The figure shows three views and two pictorial views of one solid part (mm, origin at its lowest corner). Answer the questions. A direction names the side the tool comes from. Coordinates: 2 decimals unless noted, no trailing zeros. Loops run counter-clockwise (first coordinate to the right, second up) from the corner with the lowest first, then second, coordinate; pieces in that order, holes last.
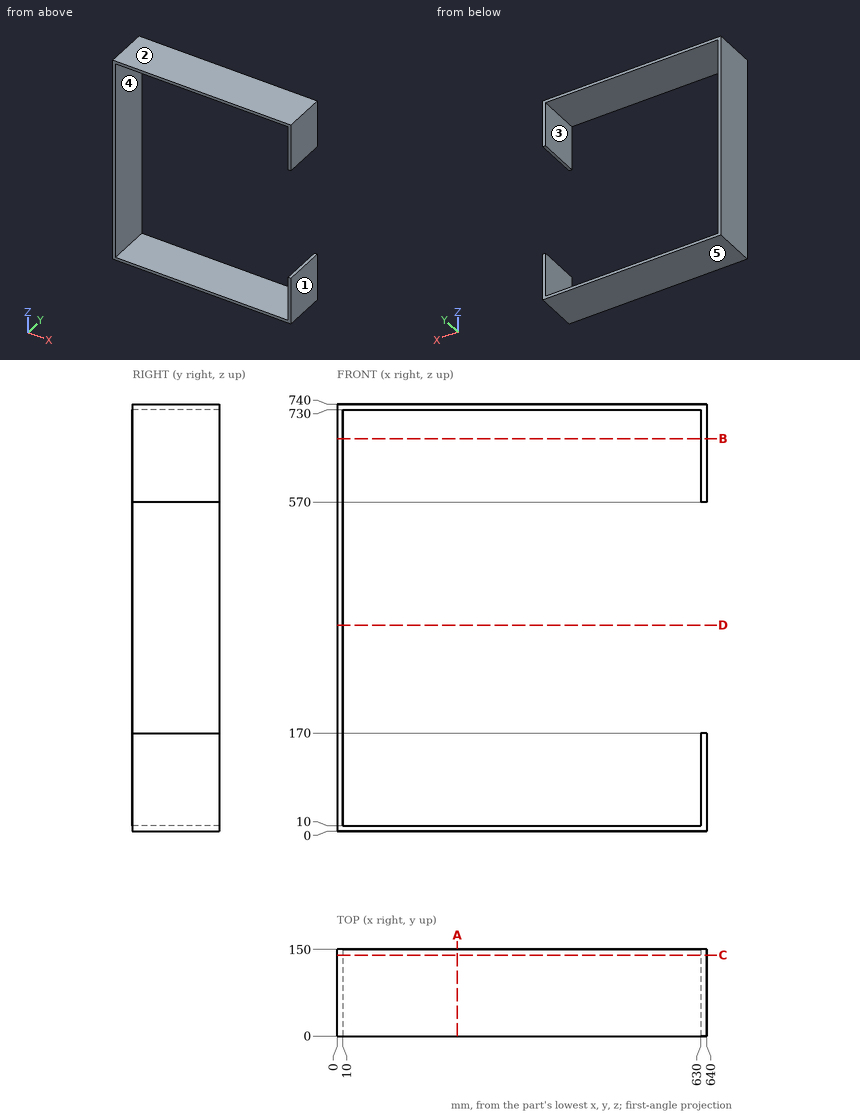
Q1. A cutting plane is placed at A-A (x = 208.5). Give the vertices of the cut face in (y, z), then the cut area to 3 significant figures.
Findings below:
outline: (0, 0) - (150, 0) - (150, 10) - (0, 10) - close; (0, 730) - (150, 730) - (150, 740) - (0, 740) - close
area: 3,000 mm2
Q2. A flat-ended cylindrical pin translates along its axis: pin 1 Ø3 at (y, z) = (65.5, 269) entering from +X. Find the tip coordinate at first contact, or state that the pin passes through.
Findings below:
pin 1: stops at x = 10
Q3. Determine the mould class of the marked faces 1, 2 and 3 for opening direction X: +X half, -X half, draft (parallel to the pull), parting line (faces both ways), or undercut.
Findings below:
face 1: +X half
face 2: draft
face 3: undercut
Q4. A cutting plane is placed at D-D (z = 357). Give the vertices of the cut face in (x, y), then the cut area to 3 significant figures.
Findings below:
outline: (0, 0) - (10, 0) - (10, 150) - (0, 150) - close
area: 1,500 mm2
Q5. Straight lines are drawn through the part: probe 1 along Z at (x, y) = (34.5, 15); probe 2 along X at (y, z) = (65.5, 39); probe 3 along X at (y, z) = (79.5, 402.5). For each, find the intervals that lie inside material, in ascending order.
Findings below:
probe 1: z = 0 to 10, 730 to 740
probe 2: x = 0 to 10, 630 to 640
probe 3: x = 0 to 10
Q6. Which of the six approach directions +Z, -Z, +X, -X, +Y, -Y give full straight-line access (tool end or side, diameter ignored) to the marked faces 4 and 5?
Findings below:
face 4: +Y, -Y
face 5: -Z, +X, -X, +Y, -Y
Q7. A cutting plane is placed at C-C (y = 140). Give the vertices of the cut face in (x, z), then the cut area to 3 significant figures.
Findings below:
outline: (0, 0) - (640, 0) - (640, 170) - (630, 170) - (630, 10) - (10, 10) - (10, 730) - (630, 730) - (630, 570) - (640, 570) - (640, 740) - (0, 740) - close
area: 23,200 mm2
Q8. A cutting plane is placed at B-B (z = 680). Give the vertices of the cut face in (x, y), then the cut area to 3 significant figures.
Findings below:
outline: (0, 0) - (10, 0) - (10, 150) - (0, 150) - close; (630, 0) - (640, 0) - (640, 150) - (630, 150) - close
area: 3,000 mm2
